Build history of the part. All positions in model axes, mm. Round coordinates to 2 decimals unless told otherwise and drop trailing zeros. Order: outer loops, then holes, each group sorted by start corner. A loop starts at its lowest first (then second) coordinate and runs counter-clockwise, first axis right, second up. Notation, with made-up numbers: (88.5, 84.5) - (144.5, 84.5) arc R19 ccw to (144.5, 104.5) - close; hole circle Ø8 at (69.5, 11.25). An arc over 180 degrees is marked (long way). Write each question's results on one line, items separated by ' | '. Start each with the question number.
```python
from build123d import *

# Parameters (mm, degrees)
F1_DEPTH = 20
F3_DEPTH = 25
F4_W     = 32.8999999911
F4_H     = 25.900002569
F5_DEPTH = 400
F6_W     = 72.2760502249
F6_H     = 60.5556070805
F7_DEPTH = 10


with BuildPart() as f1:
    # F0 (on Top) → F1 (new body)
    with BuildSketch(Plane.XY):
        with BuildLine():
            Line((0, -36.4989928704), (0, 0))
            Line((0, 0), (-36.4989928704, 0))
            ThreePointArc((-36.4989928704, 0), (-25.8086853652, -25.8086853652), (0, -36.4989928704))
        make_face()
        with BuildLine():
            Line((-36.4989928704, 0), (0, 0))
            Line((0, 0), (0, 36.4989928704))
            ThreePointArc((0, 36.4989928704), (-25.8086853652, 25.8086853652), (-36.4989928704, 0))
        make_face()
        with BuildLine():
            Line((0, 36.4989928704), (0, 0))
            Line((0, 0), (36.4989928704, 0))
            ThreePointArc((36.4989928704, 0), (25.8086853652, 25.8086853652), (0, 36.4989928704))
        make_face()
        with BuildLine():
            Line((36.4989928704, 0), (0, 0))
            Line((0, 0), (0, -36.4989928704))
            ThreePointArc((0, -36.4989928704), (25.8086853652, -25.8086853652), (36.4989928704, 0))
        make_face()
        with BuildLine():
            Line((-66.4428547025, 0), (-36.4989928704, 0))
            ThreePointArc((-36.4989928704, 0), (-25.8086853652, 25.8086853652), (0, 36.4989928704))
            Line((0, 36.4989928704), (0, 41.486993432))
            Line((0, 41.486993432), (-66.4428547025, 41.486993432))
            Line((-66.4428547025, 41.486993432), (-66.4428547025, 0))
        make_face()
        with BuildLine():
            Line((63.4185671806, 0), (36.4989928704, 0))
            ThreePointArc((36.4989928704, 0), (25.8086853652, -25.8086853652), (0, -36.4989928704))
            Line((0, -36.4989928704), (0, -44.0467298031))
            Line((0, -44.0467298031), (63.4185671806, -44.0467298031))
            Line((63.4185671806, -44.0467298031), (63.4185671806, 0))
        make_face()
    extrude(amount=F1_DEPTH)

    # F2 (on Top) → F3 (join)
    with BuildSketch(Plane.XY):
        Polygon((57.8724933064, 74.5838845975), (-36.6974943524, 55.7911281579), (-10.9426933471, 26.4123254008), (-9.5999531063, 25.5090280786), (-8.1394452782, 23.6443783888), (-4.9307275448, 27.8466683828), (1.2793188629, 32.1364451441), (8.5110378867, 34.2972554104), (16.0565384823, 34.1175840178), (23.1772144787, 31.615018454), (29.1760444968, 27.0345272727), (33.465821258, 20.824480865), (35.6266315244, 13.5927618412), (35.511328062, 8.7504642912), align=None)
        Polygon((-9.5999531063, 25.5090280786), (-10.9426933471, 26.4123254008), (-8.3148280565, 23.414688726), (-8.1394452782, 23.6443783888), align=None)
        Polygon((-8.3148280565, 23.414688726), (-10.9426933471, 26.4123254008), (-16.3222458945, 30.0312944786), (-24.1129834259, 32.2549226939), (-32.2095540295, 31.962248502), (-39.8194089626, 29.181920892), (-46.1976426034, 24.186097702), (-50.7199090034, 17.4638049138), (-52.9435372187, 9.6730673824), (-52.6508630268, 1.5764967788), (-49.8705354168, -6.0333581543), (-44.8747122268, -12.4115917951), (-38.1524194386, -16.933858195), (-30.3616819072, -19.1574864104), (-22.2651113036, -18.8648122185), (-14.6552563705, -16.0844846085), (-8.2770227297, -11.0886614185), (-5.2710709409, -6.6203514508), (-5.7428686549, -6.2601036588), (-10.0326454161, -0.0500572511), (-12.1934556825, 7.1816617728), (-12.0137842899, 14.7271623684), (-9.5112187261, 21.8478383648), align=None)
        Polygon((35.4469601318, 6.0472612456), (35.511328062, 8.7504642912), (31.5576392107, -2.889575799), (32.944394568, -1.0734147508), align=None)
        Polygon((31.5576392107, -2.889575799), (35.511328062, 8.7504642912), (35.6266315244, 13.5927618412), (33.465821258, 20.824480865), (29.1760444968, 27.0345272727), (23.1772144787, 31.615018454), (16.0565384823, 34.1175840178), (8.5110378867, 34.2972554104), (1.2793188629, 32.1364451441), (-4.9307275448, 27.8466683828), (-8.1394452782, 23.6443783888), (-4.9795485535, 19.6100963847), (22.1651728078, -11.3542047802), (28.3639033867, -7.0722447689), align=None)
        Polygon((-4.9795485535, 19.6100963847), (-8.3148280565, 23.414688726), (-9.5112187261, 21.8478383648), (-12.0137842899, 14.7271623684), (-12.1934556825, 7.1816617728), (-10.0326454161, -0.0500572511), (-5.7428686549, -6.2601036588), (-5.2710709409, -6.6203514508), (-3.7547563298, -4.3663686303), (-1.5311281144, 3.4243689011), (-1.8238023063, 11.5209395047), (-4.6041299163, 19.1307944379), align=None)
        Polygon((26.8625039607, -16.7125053704), (31.5576392107, -2.889575799), (28.3639033867, -7.0722447689), (22.1651728078, -11.3542047802), align=None)
        Polygon((22.1651728078, -11.3542047802), (-4.9795485535, 19.6100963847), (-4.6041299163, 19.1307944379), (-1.8238023063, 11.5209395047), (-1.5311281144, 3.4243689011), (-3.7547563298, -4.3663686303), (-5.2710709409, -6.6203514508), (0.2559613631, -10.84059484), (7.3766373596, -13.3431604039), (14.9221379551, -13.5228317965), (22.153856979, -11.3620215301), align=None)
    extrude(amount=F3_DEPTH)

    # F4 (on Top) → F5 (join)
    with BuildSketch(Plane.XY):
        with Locations((-40.5125012621, -39.112502709)):
            Rectangle(F4_W, F4_H)
    extrude(amount=F5_DEPTH)

    # F6 (on Top) → F7 (join)
    with BuildSketch(Plane.XY):
        with Locations((-20.344610326, -56.6111132503)):
            Rectangle(F6_W, F6_H)
    extrude(amount=F7_DEPTH)


solid = f1.part
```
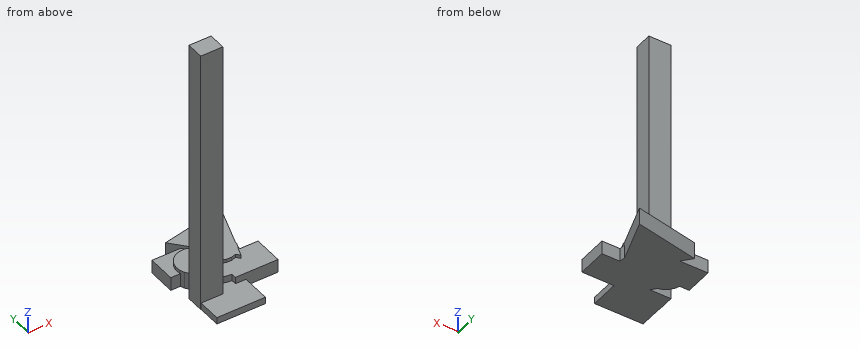
1. Cut at C-C (y = 37). List the corners of the cut face in (x, z).
2. Flat gauge pins, fed straight in: pin 1 Ø6 at (x, z) = (40, 14.5) entering from -Y; pin 2 Ø20.5 at (y, z) = (-41.5, 215) entering from -X; pin 3 Ø11 at (y, z) = (-62, 3.5) entering from +X. Where does each tip first touch, or does it go through?
3. Wall check: line 1 (Y direction, x = -52, z = 116.5); line 2 (Z direction, x = 47, y = -37.5); line 3 (Z direction, x = 19, y = 48). Give the ranges that are in metal, low to high. Write a range as from..to.
4. Cut at B-B (z = 165). List the corners of the cut face in (x, y), plus the area to 3 significant figures.
5. Cut at A-A (x = 53). List the corners of the cut face in (y, z), plus the area to 3 significant figures.
A:
1) outline: (-66.44, 0) - (45.11, 0) - (45.11, 25) - (-20.22, 25) - (-20.22, 20) - (-66.44, 20) - close
2) pin 1: stops at y = -44.05 | pin 2: stops at x = -56.96 | pin 3: stops at x = 15.79
3) line 1: y = -52.06..-26.16 | line 2: z = 0..20 | line 3: z = 0..25
4) outline: (-56.96, -52.06) - (-24.06, -52.06) - (-24.06, -26.16) - (-56.96, -26.16) - close | area: 852 mm^2
5) outline: (-44.05, 0) - (0, 0) - (0, 20) - (-44.05, 20) - close; (60.24, 0) - (73.62, 0) - (73.62, 25) - (60.24, 25) - close | area: 1,220 mm^2
